For this review, take the finished solid that the model builds, in its own axes (mm). Face numbers are marked on the shaded views. A direction names the side the tool comes from. Round coordinates to 2 decimals unless told otherwise and drop trailing zeros. Write each loop counter-clockwise with the first axis right and the second up, starting at its lowest first coordinate (ties: lowest second). Pieces come first, ordered by that corner, then holes. Notation, with made-up numbers: (-5, 28) -> (4, 28) arc R23 cw to (4, 65) -> close; hole circle Ø8 at (23, 56). An arc over 180 degrees is marked (long way). Write each question's results on one line, items separated by ' | '. Start each with the question number.
Item 1: To check wall thickness, follow line 1 along Y through (x, z) = (-48.5, 1.6); line 2 along Z through (x, y) = (-46, -20.5). State the ranges of each line that lie inside material, in increasing order.
Item 2: Clearance check with flat-ended pins moving along their axes: pin 1 (5 mm diameter, centred on x = -14.5, y = -15, fed in from +Z); pin 2 (19 mm diameter, centred on x = 0, z = 29.6, fed in from +Y); pin 3 (6.5 mm diameter, centred on x = -1, z = 18, fed in from -Y). State where each tip first meets the part, or that it passes through.
Item 3: Add section A-A (x = -18.5). State the section outline as (y, z) points.
Item 4: Add section B-B (y = 4). State the section outline as (x, z) points.
Item 5: Tool access review of the marked faces 1, 2 and 3: name each direction out of +Z, -Z, +X, -X, +Y, -Y from which nothing blocks a thin tool from reaching the whole face with its end or side.
Item 6: Add section C-C (x = 26). State the section outline as (y, z) points, plus the area to 3 significant figures.
from build123d import *

# Parameters (mm, degrees)
CROQUIS1_W              = 107
CROQUIS1_H              = 55
CROQUIS1_R              = 2
SALIENTE_EXTRUIR1_DEPTH = 2
CROQUIS2_W              = 22
CROQUIS2_H              = 2
SALIENTE_EXTRUIR2_DEPTH = 27.6
CROQUIS3_R              = 11
SALIENTE_EXTRUIR3_DEPTH = 2
CROQUIS4_R              = 6
CORTAR_EXTRUIR1_DEPTH   = 187.15
CROQUIS6_R              = 1.35
CORTAR_EXTRUIR2_DEPTH   = 187.15


with BuildPart() as part:
    # Croquis1 → Saliente-Extruir1 (new body)
    with BuildSketch(Plane.XY):
        Rectangle(CROQUIS1_W, CROQUIS1_H)
        with Locations((-48.5, 20)):
            Circle(CROQUIS1_R, mode=Mode.SUBTRACT)
        with Locations((-48.5, -20)):
            Circle(CROQUIS1_R, mode=Mode.SUBTRACT)
        with Locations((-18.5, 20)):
            Circle(CROQUIS1_R, mode=Mode.SUBTRACT)
        with Locations((-18.5, -20)):
            Circle(CROQUIS1_R, mode=Mode.SUBTRACT)
        with Locations(Location((48.5, -20, 0), (0, 0, 180))):
            Circle(CROQUIS1_R, mode=Mode.SUBTRACT)
        with Locations(Location((18.5, -20, 0), (0, 0, 180))):
            Circle(CROQUIS1_R, mode=Mode.SUBTRACT)
        with Locations(Location((18.5, 20, 0), (0, 0, 180))):
            Circle(CROQUIS1_R, mode=Mode.SUBTRACT)
        with Locations(Location((48.5, 20, 0), (0, 0, 180))):
            Circle(CROQUIS1_R, mode=Mode.SUBTRACT)
    extrude(amount=SALIENTE_EXTRUIR1_DEPTH)

    # Croquis2 → Saliente-Extruir2 (add)
    with BuildSketch(Plane(origin=(0, 0, 2), x_dir=(-1, 0, 0), z_dir=(0, 0, -1))):
        Rectangle(CROQUIS2_W, CROQUIS2_H)
    extrude(amount=-SALIENTE_EXTRUIR2_DEPTH)

    # Croquis3 → Saliente-Extruir3 (add)
    with BuildSketch(Plane(origin=(0, 1, 0), x_dir=(1, 0, 0), z_dir=(0, 1, 0))):
        with Locations((0, -29.6)):
            Circle(CROQUIS3_R)
    extrude(amount=-SALIENTE_EXTRUIR3_DEPTH)

    # Croquis4 → Cortar-Extruir1 (cut)
    with BuildSketch(Plane(origin=(0, 1, 0), x_dir=(1, 0, 0), z_dir=(0, 1, 0))):
        with Locations(Location((0, -29.6, 0), (0, 0, 270))):
            Circle(CROQUIS4_R)
    extrude(amount=-CORTAR_EXTRUIR1_DEPTH, mode=Mode.SUBTRACT)

    # Croquis6 → Cortar-Extruir2 (cut)
    with BuildSketch(Plane(origin=(0, 1, 0), x_dir=(1, 0, 0), z_dir=(0, 1, 0))):
        with Locations(Location((7.5, -29.6, 0), (0, 0, 270))):
            Circle(CROQUIS6_R)
        with Locations(Location((-3.75, -36.095190528, 0), (0, 0, 270))):
            Circle(CROQUIS6_R)
        with Locations(Location((-3.75, -23.104809472, 0), (0, 0, 270))):
            Circle(CROQUIS6_R)
    extrude(amount=-CORTAR_EXTRUIR2_DEPTH, mode=Mode.SUBTRACT)


solid = part.part
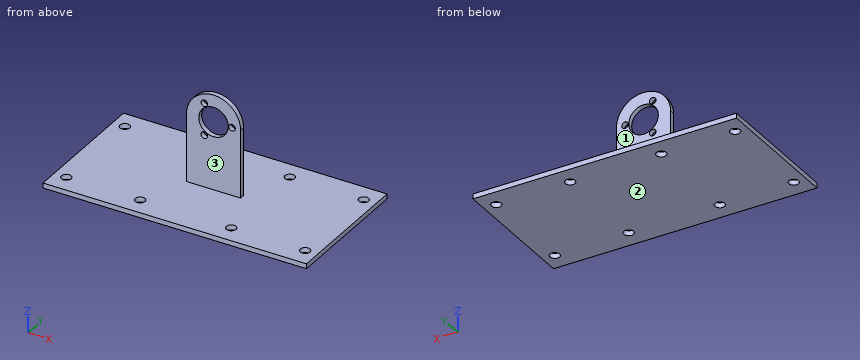
Responses:
1) line 1: y = -27.5 to -22, -18 to 18, 22 to 27.5 | line 2: z = 0 to 2
2) pin 1: stops at z = 2 | pin 2: stops at y = 1 | pin 3: stops at y = -1
3) outline: (-27.5, 0) -> (-22, 0) -> (-22, 2) -> (-27.5, 2) -> close; (-18, 0) -> (18, 0) -> (18, 2) -> (-18, 2) -> close; (22, 0) -> (27.5, 0) -> (27.5, 2) -> (22, 2) -> close
4) outline: (-53.5, 0) -> (53.5, 0) -> (53.5, 2) -> (-53.5, 2) -> close
5) face 1: +Z, +X, -X, +Y | face 2: -Z, +X, -X, +Y, -Y | face 3: +Z, +X, -X, -Y
6) outline: (-27.5, 0) -> (27.5, 0) -> (27.5, 2) -> (-27.5, 2) -> close | area: 110 mm^2
